```python
from build123d import *

# Parameters (mm, degrees)
SZKIC1_W                         = 6
SZKIC1_H                         = 2
DODANIE_WYCI_GNI_CIE1_DEPTH      = 2
SZKIC2_W                         = 8
SZKIC2_H                         = 4
WYTNIJ_WYCI_GNI_CIE1_DEPTH       = 2
WYTNIJ_WYCI_GNI_CIE2_REACH       = 8.403
SZKIC4_W                         = 1
SZKIC4_H                         = 0.3
DODANIE_WYCI_GNI_CIE2_DEPTH      = 6
DODANIE_WYCI_GNI_CIE2_DEPTH_BACK = 2.7
SZKIC3_W                         = 0.5
SZKIC3_H                         = 0.5
ZAOKR_GLENIE1_R                  = 0.1


with BuildPart() as part:
    # Szkic1 → Dodanie-wyciągnięcie1 (new body)
    with BuildSketch(Plane(origin=(0, 0, 0), x_dir=(1, 0, 0), z_dir=(0, 1, 0))):
        Rectangle(SZKIC1_W, SZKIC1_H)
    extrude(amount=DODANIE_WYCI_GNI_CIE1_DEPTH)

    # Szkic2 → Wytnij-wyciągnięcie1 (cut)
    with BuildSketch(Plane(origin=(0, 2, 0), x_dir=(1, 0, 0), z_dir=(0, 1, 0))):
        Rectangle(SZKIC2_W, SZKIC2_H)
        Polygon((2.7, 1), (3, 0.7), (3, -0.7), (2.7, -1), (1.3, -1), (1, -0.7), (0.7, -1), (-0.7, -1), (-1, -0.7), (-1.3, -1), (-2.7, -1), (-3, -0.7), (-3, 0.7), (-2.7, 1), (-1.3, 1), (-1, 0.7), (-0.7, 1), (0.7, 1), (1, 0.7), (1.3, 1), align=None, mode=Mode.SUBTRACT)
    extrude(amount=-WYTNIJ_WYCI_GNI_CIE1_DEPTH, mode=Mode.SUBTRACT)

    # Szkic4 → Wytnij-wyciągnięcie2 (cut, up to next)
    with BuildSketch(Plane.ZY.offset(3), mode=Mode.PRIVATE) as wytnij_wyci_gni_cie2_sk1:
        with Locations((0, 0.15)):
            Rectangle(SZKIC4_W, SZKIC4_H)
    wytnij_wyci_gni_cie2_tool1 = extrude(wytnij_wyci_gni_cie2_sk1.sketch, amount=-WYTNIJ_WYCI_GNI_CIE2_REACH, mode=Mode.PRIVATE) & part.part
    add(wytnij_wyci_gni_cie2_tool1.solids().sort_by_distance((-3, 0.15, 0))[0], mode=Mode.SUBTRACT)

    # Szkic3 → Dodanie-wyciągnięcie2 (add, two sides: drawn at the far end of the back side and taken through both)
    with BuildSketch(Plane(origin=(0, 0, 0), x_dir=(1, 0, 0), z_dir=(0, 1, 0)).offset(-DODANIE_WYCI_GNI_CIE2_DEPTH_BACK)):
        Rectangle(SZKIC3_W, SZKIC3_H)
        with Locations((2, 0)):
            Rectangle(SZKIC3_W, SZKIC3_H)
        with Locations((-2, 0)):
            Rectangle(SZKIC3_W, SZKIC3_H)
    extrude(amount=DODANIE_WYCI_GNI_CIE2_DEPTH + DODANIE_WYCI_GNI_CIE2_DEPTH_BACK)

    # Zaokrąglenie1
    zaokr_glenie1_edges = [part.edges().sort_by_distance(p)[0] for p in [
        (-0.25, -2.7, 0),
        (0, -2.7, -0.25),
        (0.25, -2.7, 0),
        (0, -2.7, 0.25),
        (-0.25, 6, 0),
        (0, 6, 0.25),
        (0.25, 6, 0),
        (0, 6, -0.25),
        (1.75, -2.7, 0),
        (2, -2.7, -0.25),
        (2.25, -2.7, 0),
        (2, -2.7, 0.25),
        (1.75, 6, 0),
        (2, 6, 0.25),
        (2.25, 6, 0),
        (2, 6, -0.25),
        (-2.25, -2.7, 0),
        (-2, -2.7, -0.25),
        (-1.75, -2.7, 0),
        (-2, -2.7, 0.25),
        (-2.25, 6, 0),
        (-2, 6, 0.25),
        (-1.75, 6, 0),
        (-2, 6, -0.25),
    ]]
    fillet(zaokr_glenie1_edges, radius=ZAOKR_GLENIE1_R)


solid = part.part
```
Model file for the job. Use its own axes, mm. A direction names the side the tool comes from. Round coordinates to 2 decimals unless told otherwise and drop trailing zeros. Loops run counter-clockwise (first coordinate to the right, second up) from the corner with the lowest first, then second, coordinate; pieces in that order, holes last. Notation, with made-up numbers: M -37.5,26.25 L -20.5,26.25 A14 cw -20.5,41.25 Z; hole C -16.5,83.25 d2. An arc over 180 degrees is marked long. Put each result on its own line as item: value. Start each with the question number.
Item 1: Drill centre lines: line 1 along Y through (x, z) = (1.25, 0.55); line 2 along Y through (x, z) = (-1, 0.4); line 3 along Z through (x, y) = (2.5, 0.25). Where is each one in solid material? Low to high.
Item 2: Cut at C-C (z = -0.35). List the corners of the cut face in (x, y).
Item 3: Drop flat-ended pins along their axis: P1, Ø0.6, axis at x = -2, y = -0.5, coming from the +Z side; P2, Ø0.6, axis at y = -0.5, z = 0, coming from the +X side; P3, Ø0.6, axis at x = -2, y = 4.5, coming from the -Z side. Give the stop position or say it passes through.
Item 4: Mould opens along X. For faces 3 (the face through (2, 1, 1)), 4 (the face through (-3, 1, 0)), 5 (the face through (-1, 0.3, 0)) say: released by +X, released by -X, zero draft, split by the parting line, or undercut.
Item 5: 3-axis set-ups, long thin cutter, end or side, ignore diameter. For faces 1 (the face through (2, 1, -1)), 2 (the face through (0, 2, -0.5)): which of +Z, -Z, +X, -X, +Y, -Y reach the whole face in a straight line?
Item 6: Cut at A-A (y = -0.25). List the corners of the cut face in (x, z).
Item 7: Cut at B-B (x = 2.55). List the corners of the cut face in (y, z), then the cut area to 3 significant figures.
Item 8: Cut at D-D (x = -0.85). List the corners of the cut face in (y, z), then the cut area to 3 significant figures.
Answer block:
1. line 1: 0 to 2
1. line 2: 0.3 to 2
1. line 3: -1 to -0.5, 0.5 to 1
2. outline: M -3,0.3 L 3,0.3 L 3,2 L -3,2 Z
3. P1: z = 0.25
3. P2: x = 2.25
3. P3: z = -0.25
4. face 3: zero draft
4. face 4: released by -X
4. face 5: undercut
5. face 1: -Z, +X, -X, +Y, -Y
5. face 2: +Y
6. outline: M -2.25,-0.25 L -1.75,-0.25 L -1.75,0.25 L -2.25,0.25 Z; M -0.25,-0.25 L 0.25,-0.25 L 0.25,0.25 L -0.25,0.25 Z; M 1.75,-0.25 L 2.25,-0.25 L 2.25,0.25 L 1.75,0.25 Z
7. outline: M 0,-1 L 2,-1 L 2,1 L 0,1 L 0,0.5 L 0.3,0.5 L 0.3,-0.5 L 0,-0.5 Z
7. area: 3.70 mm2
8. outline: M 0,-0.85 L 2,-0.85 L 2,0.85 L 0,0.85 L 0,0.5 L 0.3,0.5 L 0.3,-0.5 L 0,-0.5 Z
8. area: 3.10 mm2
